Autodesk Fusion 360 part; units mm, degrees
sketch "スケッチ1" plane through (0, 0, 0) normal (0, 0, 1) x (1, 0, 0)
  line L0 (0, 0) -> (20, 0)
  line L1 (20, 0) -> (20, 40)
  line L2 (20, 40) -> (0, 40)
  line L3 (0, 40) -> (0, 0)
  dimension "d1" = 20
  dimension "d2" = 40
extrude "押し出し1" add sketch "スケッチ1" along normal blind 10
sketch "スケッチ2" plane through (0, 0, 10) normal (0, 0, 1) x (-1, 0, 0)
  line L0 (0, -40) -> (0, 0)
  line L1 (0, 0) -> (-20, 0)
  line L2 (-20, 0) -> (-20, -40)
  line L3 (-20, -40) -> (0, -40)
  line L4 (0, -47.5) -> (-20, -47.5)
  line L5 (-20, -47.5) -> (-20, 7.5)
  line L6 (-20, 7.5) -> (0, 7.5)
  line L7 (0, 7.5) -> (0, -47.5)
  dimension "d5" = 55
  dimension "d6" = 7.5
extrude "押し出し2" add sketch "スケッチ2" along normal blind 3.5
sketch "スケッチ3" plane through (0, 0, 13.5) normal (0, 0, 1) x (-1, 0, 0)
  line L0 (0, 7.5) -> (-20, 7.5)
  line L1 (-20, 7.5) -> (-20, -47.5)
  line L2 (-20, -47.5) -> (0, -47.5)
  line L3 (0, -47.5) -> (0, 7.5)
  line L4 (0, 0) -> (-20, 0)
  line L5 (-20, 0) -> (-20, -40)
  line L6 (-20, -40) -> (0, -40)
  line L7 (0, -40) -> (0, 0)
  dimension "d9" = 40
extrude "押し出し3" add sketch "スケッチ3" along normal blind 27 contours L1 L3 L4 L5 L6 L7
sketch "スケッチ4" plane through (0, 0, 0) normal (0, 0, -1) x (1, 0, 0)
  line L0 (0, 0) -> (0, -40)
  line L1 (0, -40) -> (20, -40)
  line L2 (20, -40) -> (20, 0)
  line L3 (20, 0) -> (0, 0)
  circle A0 centre (10, -10) radius 3
  dimension "d12" = 6
extrude "押し出し4" add sketch "スケッチ4" along normal blind 6.5 contours A0
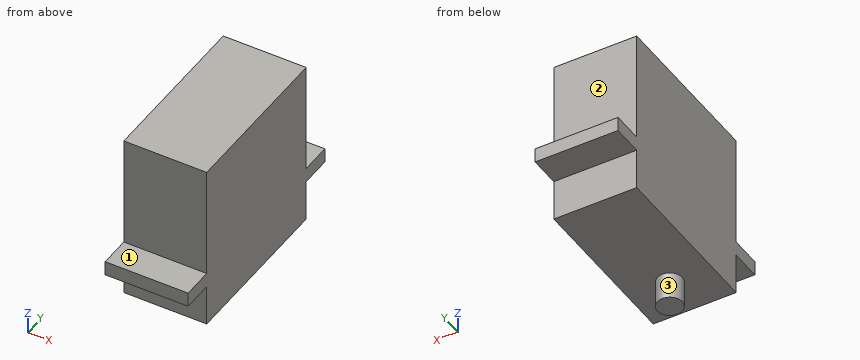
Source: CAD feature listing. Evaluate the final solid. Frame: model axes, mm. Face numbers are marked on the shaded views. A direction names the side the tool comes from. Coordinates: 2 decimals unless noted, no trailing zeros. Loops run counter-clockwise (first coordinate to the right, second up) from the corner with the lowest first, then second, coordinate; pieces in that order, holes last. Notation, with made-up numbers: (47, 28.25) -> (63, 28.25) arc R24 cw to (63, 45.25) -> close; hole circle Ø1 at (67.5, 20). An arc over 180 degrees is marked (long way). One line per item, written item: value. Start each with the question number.
Q1. Section query A-A, the plane x = 10. Return the cut outline in (y, z).
Q2. Set-up query: the marked faces 1, 2 and 3. Return all of +Z, -Z, +X, -X, +Y, -Y with unobstructed straight access to the full face (end or side cutting, diameter ignored); none if empty.
Q3. Line query: line 1 along Y through (x, z) = (18.5, 27); line 2 along Z through (x, y) = (14.75, 34); line 3 along Z through (x, y) = (5.25, -4). Output: solid intervals per line, ascending.
Q4. Section query C-C, the plane z = 9. Return the cut outline in (x, y).
Q5. Contact query for flat-ended pins moving along their axis: P1, Ø2, axis at x = 7, y = -4.5, coming from the -Z side; P2, Ø2, axis at x = 13.5, y = 44.5, coming from the +Z side; P3, Ø8, axis at x = 11, z = 5, coming from the -Y side. Output: stop coordinate, or through.
Q6. Section query D-D, the plane x = 17.25. Return the cut outline in (y, z), and give its area (3 significant figures).
Q7. Section query B-B, the plane y = 10. Return the cut outline in (x, z).
Results:
1. outline: (-7.5, 10) -> (0, 10) -> (0, 0) -> (7, 0) -> (7, -6.5) -> (13, -6.5) -> (13, 0) -> (40, 0) -> (40, 10) -> (47.5, 10) -> (47.5, 13.5) -> (40, 13.5) -> (40, 40.5) -> (0, 40.5) -> (0, 13.5) -> (-7.5, 13.5) -> close
2. face 1: +Z, +X, -X, -Y
2. face 2: +Z, +X, -X, +Y
2. face 3: -Z
3. line 1: 0 to 40
3. line 2: 0 to 40.5
3. line 3: 10 to 13.5
4. outline: (0, 0) -> (20, 0) -> (20, 40) -> (0, 40) -> close
5. P1: z = 10
5. P2: z = 13.5
5. P3: y = 0
6. outline: (-7.5, 10) -> (0, 10) -> (0, 0) -> (40, 0) -> (40, 10) -> (47.5, 10) -> (47.5, 13.5) -> (40, 13.5) -> (40, 40.5) -> (0, 40.5) -> (0, 13.5) -> (-7.5, 13.5) -> close
6. area: 1,670 mm^2
7. outline: (0, 0) -> (7, 0) -> (7, -6.5) -> (13, -6.5) -> (13, 0) -> (20, 0) -> (20, 40.5) -> (0, 40.5) -> close
